Geometry check sheet. Reference: the model listing, model coordinates, mm. A direction names the side the tool comes from. Round coordinates to 2 decimals unless told otherwise and drop trailing zeros. Loops run counter-clockwise (first coordinate to the right, second up) from the corner with the lowest first, then second, coordinate; pieces in that order, holes last. Notation, with made-up numbers: (82, 3) -> (118, 3) arc R26 ccw to (118, 37) -> close; hole circle Ø10 at (-36, 59). An arc over 180 degrees is marked (long way). Use a Markdown table: item, result. Add a question column.
Q1. Release check for a two-part mould opening along Y. For faces 1 (the face through (0, -6.605, 9)), 2 (the face through (14, 7, 10)), 3 (the face through (16, 5.395, 5)) record: released by +Y, released by -Y, zero draft, split by the parting line, or undercut.
Q2. Sectioned sample at C-C, the plane y = 2.5. Enter the section's corners in (x, z).
Q3. Set-up check for faces 4 (the face through (-2, 3.395, 9)), 5 (the face through (23.282, -7, 4)): record each of +Z, -Z, +X, -X, +Y, -Y from which the full face is reachable in a straight line by a thin tool's end or side.
Q4. Sectioned sample at D-D, the plane x = 14. Enter the section's corners in (y, z), then the cut area to 3 significant figures.
Q5. Material ranges on L1, parallel to Y at x = -1.5, z = 16.5; L2, parallel to Y at x = 20, z = 8.25; L3, parallel to X at y = 6.9, z = 7, recorded low to high.
Q6. Sectioned sample at A-A, the plane x = -1. Enter the section's corners in (y, z).
Q7. Gauge pin test, flat ends, axial feed: P1, Ø4.5, axis at x = 17, y = -7, coming from the +Z side; P2, Ø6, axis at x = 0, z = 12.5, coming from the -Y side; P3, Ø1.5, axis at y = -1, z = 2.5, coming from the +X side. Record the tip position at first contact, or that the pin passes through.
Q8. Sectioned sample at B-B, the plane z = 7. Give the number of separate pieces and of enclosed holes in the cut face, then the cut area to 3 significant figures.
Autodesk Inventor part; units mm, degrees
ref_plane "YZ Plane" through (0, 0, 0) normal (1, 0, 0) x (0, 1, 0)
ref_plane "XZ Plane" through (0, 0, 0) normal (0, 1, 0) x (-1, 0, 0)
ref_plane "XY Plane" through (0, 0, 0) normal (0, 0, 1) x (1, 0, 0)
sketch "Sketch1" plane through (0, 0, 0) normal (0, 0, 1) x (1, 0, 0)
  line L0 (-8.218, 3.3953) -> (4.282, 3.3953)
  line L1 (4.282, 3.3953) -> (4.282, -2.6047)
  line L2 (4.282, -2.6047) -> (-8.218, -2.6047)
  line L3 (-8.218, -2.6047) -> (-8.218, 3.3953)
  line L4 (-8.218, 7.3953) -> (8.282, 7.3953)
  line L5 (8.282, 7.3953) -> (8.282, -6.6047)
  line L6 (8.282, -6.6047) -> (-8.218, -6.6047)
  line L7 (-8.218, -6.6047) -> (-8.218, 7.3953)
  point P0 (0, 0)
  dimension "d0" = 12.5
  dimension "d1" = 6
  dimension "d2" = 4
  dimension "d3" = 4
  dimension "d4" = 4
extrude "Extrusion1" add sketch "Sketch1" along normal blind 18 contours L7 L4 L5 L6 L2 L1 L0
sketch "Sketch2" plane through (8.282, -6.6047, 0) normal (1, 0, 0) x (0, 0, -1)
  line L0 (-10, 12) -> (0, 12)
  line L1 (0, 12) -> (0, 2)
  line L2 (0, 2) -> (-10, 2)
  line L3 (-10, 2) -> (-10, 12)
  line L4 (0, 14) -> (0, 0)
  line L5 (0, 14) -> (-18, 14)
  line L6 (0, 0) -> (-18, 0)
  line L7 (-10, 12) -> (0, 12)
  line L8 (0, 12) -> (0, 16)
  line L9 (0, 16) -> (-10, 16)
  line L10 (-10, 16) -> (-10, 12)
  line L11 (0, 2) -> (-10, 2)
  line L12 (-10, 2) -> (-10, -2)
  line L13 (-10, -2) -> (0, -2)
  line L14 (0, -2) -> (0, 2)
  point P0 (0, 6.6047)
  dimension "d7" = 10
  dimension "d8" = 10
  dimension "d9" = 2
  dimension "d10" = 2
  dimension "d11" = 4
  dimension "d12" = 4
extrude "Extrusion2" add sketch "Sketch2" along normal blind 15 contours L10 L5 L4 L0 | L2 L4 L6 L12 | L10 L9 L8 L5 | L6 L14 L13 L12
chamfer "Chamfer1" distance 2 angle 45 1 edges at (8.282, -6.6047, 5)
chamfer "Chamfer2" distance 2 angle 45 1 edges at (8.282, 7.3953, 5)
sketch "Sketch3" plane through (23.282, 9.3953, 10) normal (0, 1, 0) x (1, 0, 0)
  line L0 (-15, 0) -> (0, 0)
  line L1 (0, 10) -> (0, 0)
  circle A0 centre (-5, 3) radius 1.25
  point P0 (-23.282, 10)
  dimension "d21" = 3
  dimension "d22" = 5
  dimension "d23" = 2.5
extrude "Extrusion3" cut sketch "Sketch3" against normal blind 30
chamfer "Chamfer3" distance 2 angle 45 4 edges at (23.282, -6.6047, 10) (23.282, 7.3953, 10) (-8.218, 5.3953, 0) (-8.218, -4.6047, 0)
chamfer "Chamfer4" distance 2 angle 45 1 edges at (8.282, 0.3953, 18)
properties part number "Bottom pully rack"
Values:
| question | item | result |
|---|---|---|
| 1 | face 1 | released by -Y |
| 1 | face 2 | zero draft |
| 1 | face 3 | undercut |
| 2 | outline | (4.28, 0) -> (8.28, 0) -> (8.28, 16) -> (6.28, 18) -> (4.28, 18) -> close |
| 3 | face 4 | +Z, -Z, -X |
| 3 | face 5 | +Z, -Z, +X, +Y, -Y |
| 4 | outline | (-8.6, 0) -> (-4.6, 0) -> (-4.6, 10) -> (-8.6, 10) -> close; (5.4, 0) -> (9.4, 0) -> (9.4, 10) -> (5.4, 10) -> close |
| 4 | area | 80.0 mm^2 |
| 5 | L1 | -6.6 to -2.6, 3.4 to 7.4 |
| 5 | L2 | -8.6 to -4.6, 5.4 to 9.4 |
| 5 | L3 | -8.22 to 17.03, 19.53 to 23.28 |
| 6 | outline | (-6.6, 0) -> (-2.6, 0) -> (-2.6, 18) -> (-6.6, 18) -> close; (3.4, 0) -> (7.4, 0) -> (7.4, 18) -> (3.4, 18) -> close |
| 7 | P1 | z = 10 |
| 7 | P2 | y = -6.6 |
| 7 | P3 | x = 8.28 |
| 8 | separate pieces | 3 |
| 8 | enclosed holes | 0 |
| 8 | area | 260 mm^2 |
